Read the model definition and answer for the solid it produces. Units are mm, in the model's axes. Face numbers are marked on the shaded views. A direction names the side the tool comes from. Coordinates: 2 decimals unless noted, no trailing zeros. Loops run counter-clockwise (first coordinate to the right, second up) from the corner with the lowest first, then second, coordinate; pieces in that order, holes last. Notation, with made-up numbers: M 67,68.25 L 106,68.25 A26 cw 106,87.25 Z; hole C 65,-37 d8. An arc over 180 degrees is marked long. Use one line per item in the form item = value. Start each with the question number.
1. The part is cut by section C-C (y = 1). Give the vertices of the cut face in (x, z), plus the area to 3 significant figures.
2. The part is cut by section B-B (x = 4.25). Give the vertices of the cut face in (y, z).
3. Find the intervals of material crossed by probe 1 along Y at (x, z) = (9.25, 13.75); probe 2 along Y at (x, z) = (12, 8.25); probe 3 along X at (y, z) = (1, 5.25), in increasing order. Write a range as [from, to].
4. For a pull along Y with two mould halves and no side action, classify the marked faces 1, 2 and 3 as released by +Y, released by -Y, zero draft, split by the parting line, or undercut.
5. Flat-ended cylindrical pins translate along their axes: pin 1 (3 mm diameter, centred on y = 11, z = 10, fed in from -X); pin 2 (1.5 mm diameter, centred on x = 6.5, y = 8, fed in from -Z); pin 3 (2 mm diameter, centred on x = -1, y = -1, fed in from +Z). Find the tip coordinate at first contact, or state that the pin passes through.
6. A tool of negligible diameter and unlimited length cuts with its end or side. For the marked faces 4, 5 and 6, from which of +Z, -Z, +X, -X, +Y, -Y can it reach the whole face along a straight path? Write none if from no direction.
7. The part is cut by section D-D (y = 8.5). Give the vertices of the cut face in (x, z), plus the area to 3 significant figures.
8. The part is cut by section A-A (z = 7). Give the vertices of the cut face in (x, y), plus the area to 3 significant figures.
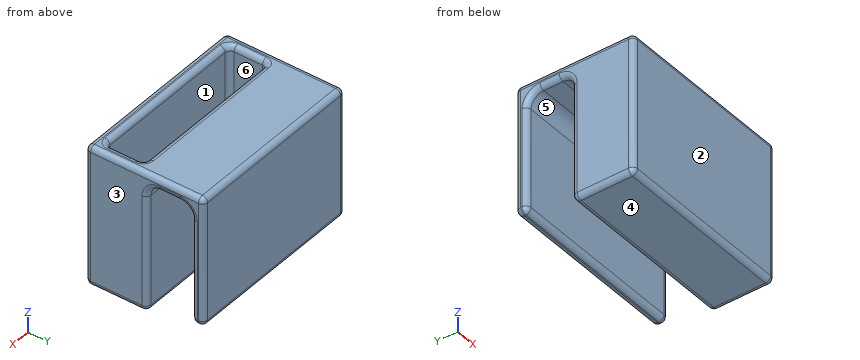
Autodesk Inventor part; units mm, degrees
ref_plane "YZ Plane" through (0, 0, 0) normal (1, 0, 0) x (0, 1, 0)
ref_plane "XZ Plane" through (0, 0, 0) normal (0, 1, 0) x (-1, 0, 0)
ref_plane "XY Plane" through (0, 0, 0) normal (0, 0, 1) x (1, 0, 0)
sketch "Sketch1" plane through (0, 0, 0) normal (0, 0, 1) x (1, 0, 0)
  line L0 (-20.02, 0) -> (20.02, 0)
  line L1 (0, -8.48) -> (0, 17.28)
  line L2 (-12.5, 3) -> (12.5, 3)
  line L3 (12.5, 3) -> (12.5, -3)
  line L4 (12.5, -3) -> (-12.5, -3)
  line L5 (-12.5, -3) -> (-12.5, 3)
  line L6 (14.3, 4.8) -> (-14.3, 4.8)
  line L7 (-14.3, 4.8) -> (-14.3, -4.8)
  line L8 (-14.3, -4.8) -> (14.3, -4.8)
  line L9 (14.3, -4.8) -> (14.3, 4.8)
  point P0 (0, 0)
  dimension "d0" = 1.8
  dimension "d1" = 25
  dimension "d2" = 6
extrude "Extrusion1" add sketch "Sketch1" along normal blind 20 contours L7 L6 L1 L2 L5 L0 | L0 L5 L4 L1 L8 L7 | L6 L9 L0 L3 L2 L1 | L1 L4 L3 L0 L9 L8
ref_plane "Work Plane1" through (0, 0, -1.8) normal (0, 0, -1) x (-1, 0, 0)
sketch "Sketch3" plane through (0, 0, -1.8) normal (0, 0, -1) x (-1, 0, 0)
  line L0 (-14.3, -4.8) -> (-14.3, 4.8)
  line L1 (-12.5, -3) -> (-12.5, 3)
  line L2 (-12.5, 3) -> (12.5, 3)
  line L3 (12.5, 3) -> (12.5, -3)
  line L4 (12.5, -3) -> (-12.5, -3)
  line L5 (-14.3, 4.8) -> (14.3, 4.8)
  line L6 (-14.3, -4.8) -> (-14.3, 4.8)
  line L7 (14.3, -4.8) -> (-14.3, -4.8)
  line L8 (14.3, 4.8) -> (14.3, -4.8)
  point P0 (0, 0)
extrude "Extrusion2" add sketch "Sketch3" against normal blind 1.8 contours L0 L5 L8 L7 | L1 L2 L3 L4
sketch "Sketch2" plane through (14.3, -4.8, 0) normal (1, 0, 0) x (0, 0, -1)
  line L0 (0, 1.8) -> (-20, 1.8)
  line L1 (1.8, 9.6) -> (-20, 9.6)
  line L2 (-20, 0) -> (-20, 9.6)
  line L3 (1.8, 0) -> (-20, 0)
  line L4 (-20, 9.6) -> (-20, 18.4)
  line L5 (-20, 18.4) -> (0, 18.4)
  line L6 (0, 18.4) -> (0, 16.6)
  line L7 (0, 16.6) -> (-18.2, 16.6)
  line L8 (-18.2, 16.6) -> (-18.2, 9.6)
  line L9 (1.8, 9.6) -> (1.8, 0)
  point P0 (0, 4.8)
  dimension "d5" = 1.8
  dimension "d6" = 1.8
  dimension "d7" = 7
extrude "Extrusion3" add sketch "Sketch2" against normal blind 28.6 contours L1 L4 L5 L6 L7 L8
fillet "Fillet1" radius 2 2 edges at (0, 4.8, 18.2) (0, 11.8, 18.2)
fillet "Fillet2" radius 0.8 33 edges at (14.3, 4.4, 20) (14.3, 13.6, 10) (14.3, 8.3, 18.2) (14.3, 11.8, 8.1) (14.3, 4.8, 7.2) (14.3, -4.8, 9.1) (14.3, 0, -1.8) (0, 4.8, -1.8) (-14.3, 8.3, 18.2) (-14.3, 11.8, 8.1) (-14.3, 4.8, 7.2) (0, 11.8, 0) (14.3, 12.7, 0) (0, 13.6, 0) (-14.3, 12.7, 0) (0, 13.6, 20) (-14.3, 13.6, 10) (-14.3, 4.4, 20) (0, -4.8, 20) (-14.3, -4.8, 9.1) (0, -4.8, -1.8) (-14.3, 0, -1.8) (0, -3, 20) (12.5, 0, 20) (0, 3, 20) (-12.5, 0, 20) (-12.5, -3, 10) (0, -3, 0) (-12.5, 0, 0) (-12.5, 3, 10) (0, 3, 0) (12.5, -3, 10) (12.5, 3, 10)
properties part number "sd.adapter"
Computed values:
q1.outline = M -14.3,-1 A0.8 ccw -13.5,-1.8 L 13.5,-1.8 A0.8 ccw 14.3,-1 L 14.3,19.2 A0.8 ccw 13.5,20 L 13.3,20 A0.8 ccw 12.5,19.2 L 12.5,0 L -11.7,0 A0.8 cw -12.5,0.8 L -12.5,19.2 A0.8 ccw -13.3,20 L -13.5,20 A0.8 ccw -14.3,19.2 Z
q1.area = 123 mm²
q2.outline = M -4.8,-1 A0.8 ccw -4,-1.8 L 4,-1.8 A0.8 ccw 4.8,-1 L 4.8,16.2 A2 cw 6.8,18.2 L 9.8,18.2 A2 cw 11.8,16.2 L 11.8,0.8 A0.8 ccw 12.6,0 L 12.8,0 A0.8 ccw 13.6,0.8 L 13.6,19.2 A0.8 ccw 12.8,20 L 3.8,20 A0.8 ccw 3,19.2 L 3,0.8 A0.8 cw 2.2,0 L -2.2,0 A0.8 cw -3,0.8 L -3,19.2 A0.8 ccw -3.8,20 L -4,20 A0.8 ccw -4.8,19.2 Z
q3.probe_1 = [-4.8, -3], [3, 4.8], [11.8, 13.6]
q3.probe_2 = [-4.8, -2.94], [2.94, 4.8], [11.8, 13.6]
q3.probe_3 = [-14.3, -12.5], [12.5, 14.3]
q4.face_1 = undercut
q4.face_2 = released by -Y
q4.face_3 = zero draft
q5.pin_1 = -14.29
q5.pin_2 = 18.2
q5.pin_3 = 0
q6.face_4 = -Z, +X, -X, +Y, -Y
q6.face_5 = -Z, +X, -X
q6.face_6 = +Z
q7.outline = M -14.3,19 A0.8 ccw -13.5,18.2 L 13.5,18.2 A0.8 ccw 14.3,19 L 14.3,19.2 A0.8 ccw 13.5,20 L -13.5,20 A0.8 ccw -14.3,19.2 Z
q7.area = 50.9 mm²
q8.outline = M -14.3,-4 A0.8 ccw -13.5,-4.8 L 13.5,-4.8 A0.8 ccw 14.3,-4 L 14.3,4 A0.8 ccw 13.5,4.8 L -13.5,4.8 A0.8 ccw -14.3,4 Z; M -14.3,12.6 A0.8 ccw -13.5,11.8 L 13.5,11.8 A0.8 ccw 14.3,12.6 L 14.3,12.8 A0.8 ccw 13.5,13.6 L -13.5,13.6 A0.8 ccw -14.3,12.8 Z; hole M -12.5,-2.2 A0.8 ccw -11.7,-3 L 11.7,-3 A0.8 ccw 12.5,-2.2 L 12.5,2.2 A0.8 ccw 11.7,3 L -11.7,3 A0.8 ccw -12.5,2.2 Z
q8.area = 175 mm²
